from build123d import *

# Parameters (mm, degrees)
COQUE1_T                     = 2.5
ENL_V_MAT_EXTRU_1_DEPTH      = 20.052558883
ENL_V_MAT_EXTRU_1_DEPTH_BACK = 20.052558883
ESQUISSE2_R                  = 2
ESQUISSE3_R                  = 3.5
ESQUISSE3_R_2                = 2
EXTRU_MINCE1_DEPTH           = 21
CONG_1_R                     = 7
ENL_V_MAT_EXTRU_2_DEPTH      = 27.057628564
ENL_V_MAT_EXTRU_2_DEPTH_BACK = 27.057628564
ESQUISSE5_R                  = 0.5


with BuildPart() as part:
    # Esquisse1 → Révolution1 (revolve)
    with BuildSketch(Plane.XY):
        with BuildLine():
            Line((-11, 0), (11, 0))
            ThreePointArc((11, 0), (0, 11), (-11, 0))
        make_face()
    revolve(axis=Axis((-11, 0, 0), (1, 0, 0)))

    # Coque1 (no face opened: a closed hollow body)
    add(offset(amount=-COQUE1_T, mode=Mode.PRIVATE), mode=Mode.SUBTRACT)

    # Esquisse2 → Enlèv. mat.-Extru.1 (cut, two sides: drawn at the far end of the back side and taken through both)
    with BuildSketch(Plane(origin=(0, 0, 0), x_dir=(1, 0, 0), z_dir=(0, 1, 0)).offset(-ENL_V_MAT_EXTRU_1_DEPTH_BACK)):
        with Locations(Location((0, 0, 0), (0, 0, 270))):
            Circle(ESQUISSE2_R)
    extrude(amount=ENL_V_MAT_EXTRU_1_DEPTH + ENL_V_MAT_EXTRU_1_DEPTH_BACK, mode=Mode.SUBTRACT)

    # Esquisse3 → Extru.-Mince1 (add)
    with BuildSketch(Plane(origin=(0, 0, 0), x_dir=(0, 0, -1), z_dir=(1, 0, 0))):
        Circle(ESQUISSE3_R)
        Circle(ESQUISSE3_R_2, mode=Mode.SUBTRACT)
    extrude(amount=EXTRU_MINCE1_DEPTH)

    # Congé1
    cong_1_edges = [part.edges().sort_by_distance(p)[0] for p in [
        (10.428326807, -2.474873734, 2.474873734),
    ]]
    fillet(cong_1_edges, radius=CONG_1_R)

    # Esquisse4 → Révolution4 (revolve)
    with BuildSketch(Plane.XY):
        with BuildLine():
            Line((-9.287174866, 5.894775909), (-12.493705663, 0.842910886))
            ThreePointArc((-12.493705663, 0.842910886), (-12.666967343, 0.460123427), (-12.727263641, 0.044298698))
            Line((-12.727263641, 0.044298698), (-9.307579549, 0.032396096))
            Line((-9.307579549, 0.032396096), (-9.287174866, 5.894775909))
        make_face()
    revolve(axis=Axis((-9.307579549, 0.032396096, 0), (-0.9999939427166084, 0.00348059335354882, 0)))

    # Esquisse5 → Enlèv. mat.-Extru.2 (cut, two sides: drawn at the far end of the back side and taken through both)
    with BuildSketch(Plane(origin=(0, 0, 0), x_dir=(1, 0, 0), z_dir=(0, 1, 0)).offset(-ENL_V_MAT_EXTRU_2_DEPTH_BACK)):
        with Locations(Location((18, 0, 0), (0, 0, 270))):
            Circle(ESQUISSE5_R)
    extrude(amount=ENL_V_MAT_EXTRU_2_DEPTH + ENL_V_MAT_EXTRU_2_DEPTH_BACK, mode=Mode.SUBTRACT)


solid = part.part
Source: CAD feature listing. Evaluate the final solid. Frame: model axes, mm. A direction names the side the tool comes from. Round coordinates to 2 decimals unless told otherwise and drop trailing zeros. Loops run counter-clockwise (first coordinate to the right, second up) from the corner with the lowest first, then second, coordinate; pieces in that order, holes last. Notation, with made-up numbers: (-27, -26) - (-18, -26) arc R3 ccw to (-18, -21) - close; hole circle Ø5 at (-40, 61.25). An arc over 180 degrees is marked (long way). Write item = value, one per line. Start each with the question number.
Item 1: Section query B-B on x = 3. Output: boundary loops of the cut face in (y, z).
Item 2: Mould query, pull axis Y, two halves, no side actions, for faces 1 (the face through (17.765, -1.341, -3.233)), 2 (the face through (3.819, -1.341, -3.233)), 3 (the face through (18.496, -2.729, -0.065)). Classes: released by +Y, released by -Y, zero draft, split by the parting line, or undercut.
Item 3: Reachability of faces 4 (the face through (15.837, -0.766, -1.847)), 5 (the face through (-2, -10, 0)), 6 (the face through (-2, 10, 0)), 7 (the face through (4, -2, 0)), 8 (the face through (18.496, 2.707, -0.065)) from +Z, -Z, +X, -X, +Y, -Y: full face, straight path, thin tool, end or side. Return the list, or none.
Item 4: First-contact query: pin 1 Ø6.5 at (x, z) = (0, 0) entering from -Y; pin 2 Ø6 at (x, y) = (16.5, -4) entering from +Z; pin 3 Ø3 at (x, z) = (-2.5, 6.5) entering from +Y; pin 4 Ø1.5 at (y, z) = (-5, -3.5) entering from +X. Flat tips, straight axial feed; report the tip coordinate or a pass-through.
Item 5: Material intervals for line 1 (Y direction, x = 7, z = 1.25); line 2 (Y direction, x = 5.25, z = 0); line 3 (Z direction, x = -7.5, y = -2), sorted ascending.
Item 6: Section query C-C on y = 7.5. Output: boundary loops of the cut face in (x, z).
Results list:
q1.outline = circle Ø21.17 at (0, 0); circle Ø7 at (0, 0); hole circle Ø15.91 at (0, 0); hole circle Ø4 at (0, 0)
q2.face_1 = split by the parting line
q2.face_2 = undercut
q2.face_3 = zero draft
q3.face_4 = +X
q3.face_5 = -Y
q3.face_6 = +Y
q3.face_7 = none
q3.face_8 = +Y, -Y
q4.pin_1 = -10.82
q4.pin_2 = 3.35
q4.pin_3 = 9.55
q4.pin_4 = 9.88
q5.line_1 = -8.39 to -4.66, -3.27 to -1.56, 1.56 to 3.27, 4.66 to 8.39
q5.line_2 = -9.67 to -6.68, -3.5 to -2, 2 to 3.5, 6.68 to 9.67
q5.line_3 = -7.79 to -3.46, 3.46 to 7.79
q6.outline = circle Ø16.09 at (0, 0); hole circle Ø8 at (0, 0)
